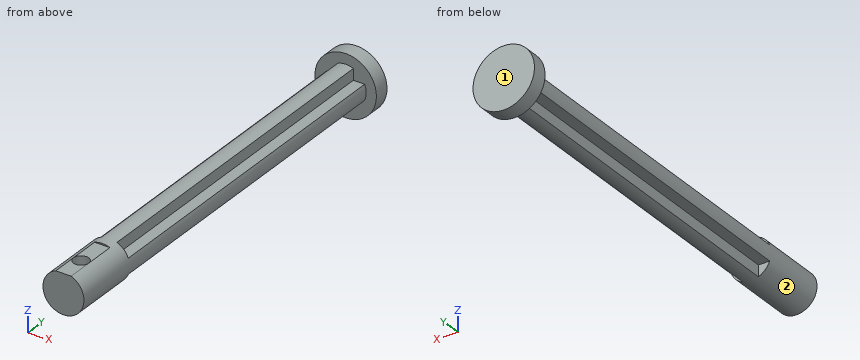
from build123d import *

# Parameters (mm, degrees)
SKETCH1_R           = 4
BOSS_EXTRUDE1_DEPTH = 80
CUT_EXTRUDE1_DEPTH  = 11
SKETCH3_R           = 1.5
CUT_EXTRUDE2_DEPTH  = 4
CUT_EXTRUDE3_DEPTH  = 67
SKETCH5_R           = 6
BOSS_EXTRUDE2_DEPTH = 3


with BuildPart() as part:
    # Sketch1 → Boss-Extrude1 (new body)
    with BuildSketch(Plane(origin=(0, 0, 0), x_dir=(1, 0, 0), z_dir=(0, 1, 0))):
        Circle(SKETCH1_R)
    extrude(amount=BOSS_EXTRUDE1_DEPTH)

    # Sketch2 → Cut-Extrude1 (cut)
    with BuildSketch(Plane.XZ):
        with BuildLine():
            Line((-1.5, 3.708099244), (1.5, 3.708099244))
            ThreePointArc((1.5, 3.708099244), (0, 4), (-1.5, 3.708099244))
        make_face()
    extrude(amount=-CUT_EXTRUDE1_DEPTH, mode=Mode.SUBTRACT)

    # Sketch3 → Cut-Extrude2 (cut)
    with BuildSketch(Plane.XY.offset(3.708099244)):
        with Locations((0, 5)):
            Circle(SKETCH3_R)
    extrude(amount=-CUT_EXTRUDE2_DEPTH, mode=Mode.SUBTRACT)

    # Sketch4 → Cut-Extrude3 (cut)
    with BuildSketch(Plane(origin=(0, 80, 0), x_dir=(1, 0, 0), z_dir=(0, 1, 0))):
        with BuildLine():
            Line((-1.5, -3.586397938), (-1.5, -3.708099244))
            ThreePointArc((-1.5, -3.708099244), (-2.828427125, -2.828427125), (-3.708099244, -1.5))
            Line((-3.708099244, -1.5), (-1.5, -1.5))
            Line((-1.5, -1.5), (-1.5, -3.586397938))
        make_face()
        with BuildLine():
            Line((-3.708099244, 1.5), (-1.5, 1.5))
            Line((-1.5, 1.5), (-1.5, 3.708099244))
            ThreePointArc((-1.5, 3.708099244), (-2.828427125, 2.828427125), (-3.708099244, 1.5))
        make_face()
        with BuildLine():
            Line((1.5, 3.708099244), (1.5, 1.5))
            Line((1.5, 1.5), (3.708099244, 1.5))
            ThreePointArc((3.708099244, 1.5), (2.828427125, 2.828427125), (1.5, 3.708099244))
        make_face()
        with BuildLine():
            Line((1.5, -3.708099244), (1.5, -1.5))
            Line((1.5, -1.5), (3.708099244, -1.5))
            ThreePointArc((3.708099244, -1.5), (2.828427125, -2.828427125), (1.5, -3.708099244))
        make_face()
    extrude(amount=-CUT_EXTRUDE3_DEPTH, mode=Mode.SUBTRACT)

    # Sketch5 → Boss-Extrude2 (add)
    with BuildSketch(Plane(origin=(0, 80, 0), x_dir=(1, 0, 0), z_dir=(0, 1, 0))):
        Circle(SKETCH5_R)
    extrude(amount=BOSS_EXTRUDE2_DEPTH)


solid = part.part
Geometry: final body of the model. Coordinates: model frame, mm. Face numbers are marked on the shaded views. A direction names the side the tool comes from. Give positions to 0.01 mm unless a question says otherwise; leave off trailing zeros. Order: outer loops, then holes, each group sorted by start corner. A loop starts at its lowest first (then second) coordinate and runs counter-clockwise, first axis right, second up. Notation, with made-up numbers: (3.5, 30) -> (21.5, 30) arc R18 cw to (21.5, 37) -> close; hole circle Ø3 at (89, 63). An arc over 180 degrees is marked (long way). Write each question's results on one line, items separated by ' | '.
1) Cut plane A-A (x = 0). Output: boundary loops of the cut face in (y, z), and give its area (3 significant figures).
Geometry says:
outline: (0, -4) -> (80, -4) -> (80, -6) -> (83, -6) -> (83, 6) -> (80, 6) -> (80, 4) -> (11, 4) -> (11, 3.71) -> (6.5, 3.71) -> (6.5, -0.29) -> (3.5, -0.29) -> (3.5, 3.71) -> (0, 3.71) -> close | area: 661 mm²
2) First-contact query: pin 1 Ø3.5 at (x, y) = (0, 5) entering from +Z; pin 2 Ø1.8 at (x, y) = (3, 30.5) entering from -Z; pin 3 Ø5 at (x, y) = (0, 5) entering from -Z. Flat tips, straight axial feed; report the tip coordinate or a pass-through.
Geometry says:
pin 1: stops at z = 3.71 | pin 2: stops at z = -1.5 | pin 3: stops at z = -4
3) Set-up query: the marked faces 1 and 2. Return all of +Z, -Z, +X, -X, +Y, -Y with unobstructed straight access to the full face (end or side cutting, diameter ignored); none if empty.
Geometry says:
face 1: +Z, -Z, +X, -X, +Y | face 2: -Y
4) Line query: line 1 along Y through (x, z) = (0, 1.45); line 2 along Z through (x, y) = (2.5, 53.5); line 3 along Y through (x, z) = (3, 2.5). Output: solid intervals per line, ascending.
Geometry says:
line 1: y = 0 to 3.5, 6.5 to 83 | line 2: z = -1.5 to 1.5 | line 3: y = 0 to 13, 80 to 83
5) Cut plane B-B (y = 55.5). Output: boundary loops of the cut face in (x, z).
Geometry says:
outline: (-3.71, -1.5) -> (-1.5, -1.5) -> (-1.5, -3.71) arc R4 ccw to (1.5, -3.71) -> (1.5, -1.5) -> (3.71, -1.5) arc R4 ccw to (3.71, 1.5) -> (1.5, 1.5) -> (1.5, 3.71) arc R4 ccw to (-1.5, 3.71) -> (-1.5, 1.5) -> (-3.71, 1.5) arc R4 ccw to start
